The model under review builds one solid part; all positions refer to its coordinate system, in mm. Face numbers are marked on the shaded views. A direction names the side the tool comes from. Coordinates: 2 decimals unless noted, no trailing zeros. Order: outer loops, then holes, each group sorted by start corner. A loop starts at its lowest first (then second) coordinate and runs counter-clockwise, first axis right, second up.
```python
from build123d import *

# Parameters (mm, degrees)
F3_D     = 2.2606
F3_DEPTH = 5.715
F3_TIP   = 0.6791527577
F4_R     = 5.1689
F5_DEPTH = 4.064
F6_R     = 4.0005
F7_DEPTH = 2.8702
F9_DEPTH = 25.4
F11_D    = 2.5


with BuildPart() as f1:
    # F0 (on Front) → F1 (revolve)
    with BuildSketch(Plane.XZ):
        Polygon((14.330415332, -12.5857), (14.330415332, 0), (13.314415332, 0), (13.314415332, -4.7625), (0, -4.7625), (0, -12.5857), align=None)
    revolve(axis=Axis((0, 0, -8.6741), (0, 0, 1)))

    # F3
    with Locations(Plane.XY.offset(-4.7625)):
        with Locations((9.525, 0), (-4.7625, 8.248891971), (-4.7625, -8.248891971)):
            Hole(F3_D / 2, depth=F3_DEPTH)
            with Locations((0, 0, -(F3_DEPTH + F3_TIP / 2))):  # 118° drill point
                Cone(0, F3_D / 2, F3_TIP, mode=Mode.SUBTRACT)

    # F4 (on face) → F5 (cut)
    with BuildSketch(Plane.XY.offset(-4.7625)):
        with Locations((-5.08, 0)):
            Circle(F4_R)
    extrude(amount=-F5_DEPTH, mode=Mode.SUBTRACT)

    # F6 (on face) → F7 (cut)
    with BuildSketch(Plane.XY.offset(-8.8265)):
        with Locations((-5.08, 0)):
            Circle(F6_R)
    extrude(amount=-F7_DEPTH, mode=Mode.SUBTRACT)

    # F8 (on face) → F9 (cut)
    with BuildSketch(Plane.XY.offset(-8.8265)):
        with BuildLine():
            ThreePointArc((-10.109904504, -1.190625), (-10.2489, 0), (-10.109904504, 1.190625))
            Line((-10.109904504, 1.190625), (-15.529622134, 1.190625))
            Line((-15.529622134, 1.190625), (-15.529622134, -1.190625))
            Line((-15.529622134, -1.190625), (-10.109904504, -1.190625))
        make_face()
    extrude(amount=F9_DEPTH, mode=Mode.SUBTRACT)

    # F11 (through all)
    with Locations(Plane.XY.offset(-4.7625)):
        with Locations((6.2419385775, 4.370652445)):
            Hole(F11_D / 2)


solid = f1.part
```
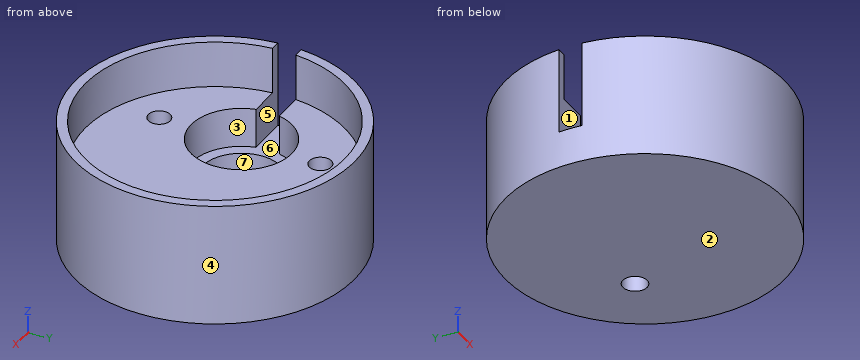
(1) We need section A-A, the plane y = -10. Write out the cut boundary in (x, z), and give its area (3 significant figures).
A:
outline: (-10.26, -12.59) - (10.26, -12.59) - (10.26, 0) - (8.79, 0) - (8.79, -4.76) - (-8.79, -4.76) - (-8.79, 0) - (-10.26, 0) - close
area: 175 mm2
(2) For pin 1 Ø4 at (x, y) = (-3.5, 1.5) entering from +Z; pin 2 Ø1.3 at (x, z) = (-12, -3) entering from +Y; pin 3 Ø2 at (x, y) = (-4.76, -8.25) entering from +Z; pin 4 Ø3 at (x, y) = (6.24, 4.37) entering from -Z, all flat-tipped, find the tip position at first contact; note any pin that passes through.
A:
pin 1: stops at z = -8.83
pin 2: stops at y = 8.75
pin 3: stops at z = -10.55
pin 4: stops at z = -12.59
(3) We need section B-B, the plane x = -7.75. Write out the cut boundary in (y, z), and give its area (3 significant figures).
A:
outline: (-12.05, -12.59) - (12.05, -12.59) - (12.05, 0) - (10.83, 0) - (10.83, -4.76) - (4.43, -4.76) - (4.43, -8.83) - (2.98, -8.83) - (2.98, -11.7) - (-2.98, -11.7) - (-2.98, -8.83) - (-4.43, -8.83) - (-4.43, -4.76) - (-10.83, -4.76) - (-10.83, 0) - (-12.05, 0) - close
area: 147 mm2
(4) Wall thickness on probe 1 along Y at (x, z) = (-5.08, -9.8); probe 2 along Z at (x, y) = (-8.25, -9.5); probe 3 along Y at (x, z) = (-9.25, -5): over which ranges is each line inside the solid? List them lowest first.
A:
probe 1: y = -13.4 to -9.33, -7.16 to -4, 4 to 7.16, 9.33 to 13.4
probe 2: z = -12.59 to -4.76
probe 3: y = -10.95 to -3.05, 3.05 to 10.95
(5) Draft analysis for pull direction X (two halves, no side actions). For the marked faces 4, 5, 6 and 7, state which applies: released by +X, released by -X, zero draft, split by the parting line, or undercut.
A:
face 4: split by the parting line
face 5: zero draft
face 6: undercut
face 7: undercut
(6) Machinability: for the marked faces 1, 2 and 3, which of the approach directions +Z, -Z, +X, -X, +Y, -Y give a long, thin tool a straight path to every point of the face, cutting with its end or side? Answer none if there is none.
A:
face 1: +Z, -X
face 2: -Z, +X, -X, +Y, -Y
face 3: +Z
(7) We need section C-C, the plane z = -4.25. Write out the cut boundary in (x, y), and give its area (3 significant figures).
A:
outline: (-14.28, -1.19) arc R14.33 ccw (long way) to (-14.28, 1.19) - (-13.26, 1.19) arc R13.31 cw (long way) to (-13.26, -1.19) - close
area: 85.8 mm2
